```python
from build123d import *

# Parameters (mm, degrees)
BOSS_EXTRUDE2_DEPTH    = 6
FILLET1_R              = 1
LPATTERN1_COUNT        = 3
LPATTERN1_PITCH        = 37.5
FILLET1_OF_LPATTERN1_R = 1
SKETCH3_W              = 6
SKETCH3_H              = 12
BOSS_EXTRUDE3_DEPTH    = 6
SKETCH4_W              = 8
SKETCH4_H              = 6
CUT_EXTRUDE2_DEPTH     = 7
LPATTERN2_COUNT        = 2
LPATTERN2_PITCH        = 37.5
BOSS_EXTRUDE4_START    = -112.5
SKETCH3_2_W            = 6
SKETCH3_2_H            = 12
BOSS_EXTRUDE4_DEPTH    = 6
SKETCH5_W              = 6
SKETCH5_H              = 22.5
BOSS_EXTRUDE5_DEPTH    = 6


with BuildPart() as part:
    # Sketch2 → Boss-Extrude2 (new body)
    with BuildSketch(Plane(origin=(0, 0, 0), x_dir=(0, 0, -1), z_dir=(1, 0, 0))):
        Polygon((-18.75, 105.5), (-18.75, 89.5), (-18.75, -89.5), (18.75, -89.5), (18.75, 89.5), (18.75, 105.5), (12, 105.5), (11, 95.5), (4, 95.5), (4, 89.5), (-4, 89.5), (-4, 95.5), (-11, 95.5), (-12, 105.5), align=None)
    boss_extrude2 = extrude(amount=BOSS_EXTRUDE2_DEPTH)

    # Fillet1
    fillet1_edges = [part.edges().sort_by_distance(p)[0] for p in [
        (3, 95.5, -4),
        (3, 105.5, -12),
        (3, 105.5, 12),
        (3, 95.5, 4),
        (3, 89.5, 4),
        (3, 89.5, -4),
    ]]
    fillet(fillet1_edges, radius=FILLET1_R)

    # LPattern1: Boss-Extrude2 ×3
    with Locations(*[(0, 0, i * LPATTERN1_PITCH) for i in range(1, LPATTERN1_COUNT)]):
        add(boss_extrude2)

    # Fillet1 of LPattern1
    fillet1_of_lpattern1_edges = [part.edges().sort_by_distance(p)[0] for p in [
        (3, 95.5, 33.5),
        (3, 105.5, 25.5),
        (3, 105.5, 49.5),
        (3, 95.5, 41.5),
        (3, 89.5, 41.5),
        (3, 89.5, 33.5),
        (3, 95.5, 71),
        (3, 105.5, 63),
        (3, 105.5, 87),
        (3, 95.5, 79),
        (3, 89.5, 79),
        (3, 89.5, 71),
    ]]
    fillet(fillet1_of_lpattern1_edges, radius=FILLET1_OF_LPATTERN1_R)

    # Sketch3 → Boss-Extrude3 (add)
    with BuildSketch(Plane(origin=(0, 0, -18.75), x_dir=(-1, 0, 0), z_dir=(0, 0, -1))):
        with Locations((-3, 79.5)):
            Rectangle(SKETCH3_W, SKETCH3_H)
        with Locations((-3, -63.5)):
            Rectangle(SKETCH3_W, SKETCH3_H)
        with Locations((-3, 8)):
            Rectangle(SKETCH3_W, SKETCH3_H)
    extrude(amount=BOSS_EXTRUDE3_DEPTH)

    # Sketch4 → Cut-Extrude2 (cut, through all)
    with BuildSketch(Plane(origin=(0, 0, 0), x_dir=(0, 0, -1), z_dir=(1, 0, 0))):
        with Locations((-18.75, 86.5)):
            Rectangle(SKETCH4_W, SKETCH4_H)
    cut_extrude2 = extrude(amount=CUT_EXTRUDE2_DEPTH, mode=Mode.SUBTRACT)

    # LPattern2: Cut-Extrude2 ×2
    with Locations(*[(0, 0, i * LPATTERN2_PITCH) for i in range(1, LPATTERN2_COUNT)]):
        add(cut_extrude2, mode=Mode.SUBTRACT)

    # Sketch3_2 → Boss-Extrude4 (add)
    with BuildSketch(Plane(origin=(0, 0, -18.75), x_dir=(-1, 0, 0), z_dir=(0, 0, -1)).offset(BOSS_EXTRUDE4_START)):
        with Locations((-3, 79.5)):
            Rectangle(SKETCH3_2_W, SKETCH3_2_H)
        with Locations((-3, -63.5)):
            Rectangle(SKETCH3_2_W, SKETCH3_2_H)
        with Locations((-3, 8)):
            Rectangle(SKETCH3_2_W, SKETCH3_2_H)
    extrude(amount=-BOSS_EXTRUDE4_DEPTH)

    # Sketch5 → Boss-Extrude5 (add)
    with BuildSketch(Plane.XZ.offset(89.5)):
        with Locations((3, 15)):
            Rectangle(SKETCH5_W, SKETCH5_H)
        with Locations((3, 60)):
            Rectangle(SKETCH5_W, SKETCH5_H)
    extrude(amount=BOSS_EXTRUDE5_DEPTH)


solid = part.part
```
The listing builds one solid part. Answer for the finished solid, in the listing's coordinates (mm). A direction names the side the tool comes from. Give positions to 0.01 mm unless a question says otherwise; leave off trailing zeros. Write each loop counter-clockwise with the first axis right and the second up, starting at its lowest first coordinate (ties: lowest second). Pieces come first, ordered by that corner, then holes. Notation, with made-up numbers: (-29.5, 54) -> (-6.5, 54) arc R6 cw to (-6.5, 62) -> close; hole circle Ø6 at (-26, -6.5). An arc over 180 degrees is marked (long way). Use one line per item in the form item = value.
1) Section A-A on z = 56 is taken. Write down the section's boundary in (x, y), plus the area to 3 significant figures.
Result:
outline = (0, -95.5) -> (6, -95.5) -> (6, 83.5) -> (0, 83.5) -> close; (0, 89.5) -> (6, 89.5) -> (6, 105.5) -> (0, 105.5) -> close
area = 1,170 mm²
2) A tool of negligible diameter and unlimited length cuts with its end or side. For faces 4 (the flat face through (3, 105.5, -16)), 5 (the flat face through (3, -57.5, 97)), 6 (the flat face through (3, 83.5, 56)), 7 (the flat face through (2.96, 99.99, 48.95)), 8 (the flat face through (6, 6, 38)), from which of +Z, -Z, +X, -X, +Y, -Y can it reach the whole face along a straight path? Write none if from no direction.
Result:
face_4 = +Z, -Z, +X, -X, +Y
face_5 = +Z, +X, -X
face_6 = +X, -X
face_7 = +X, -X, +Y
face_8 = +Z, -Z, +X, +Y, -Y
3) Section B-B on x = 2.5 is taken. Count the separate pieces of the cut face and the enclosed holes in it, plus the area to 3 significant figures.
Result:
separate_pieces = 1
enclosed_holes = 2
area = 21,700 mm²
4) Each of these flat-tipped pins is pushed along its axis until it touches: P1, Ø2, axis at x = 4.5, y = -11.5, coming from the -Z side; P2, Ø3, axis at x = 1.5, z = 33.5, coming from the -Y side; P3, Ø1.5, axis at x = 2.5, y = -30.5, coming from the +Z side. Where does it stop, or does it pass through?
Result:
P1 = -18.75
P2 = -89.5
P3 = 93.75
5) Straight lines are drawn through the part: probe 1 along Y at (x, z) = (3.6, 59.5); probe 2 along Z at (x, y) = (1.8, 1); probe 3 along Y at (x, z) = (5.25, 44.5). For each, find the intervals that lie inside material, in ascending order.
Result:
probe_1 = -95.5 to 83.5, 89.5 to 105.5
probe_2 = -18.75 to 93.75
probe_3 = -89.5 to 95.5
6) Section C-C on y = 68 is taken. Write down the section's boundary in (x, z), plus the area to 3 significant figures.
Result:
outline = (0, -18.75) -> (6, -18.75) -> (6, 93.75) -> (0, 93.75) -> close
area = 675 mm²
7) Section D-D on z = -1 is taken. Write down the section's boundary in (x, y), plus the area to 3 significant figures.
Result:
outline = (0, -89.5) -> (6, -89.5) -> (6, 89.5) -> (0, 89.5) -> close
area = 1,070 mm²
8) For a pull along Z with two mould halves and no side action, classify faces 1 (the flat face through (3, -92, 3.75)), 2 (the flat face through (3, 14, -22)), 3 (the flat face through (3, 95.5, 45)) as +Z half, -Z half, draft (parallel to the pull), parting line (faces both ways), or undercut.
Result:
face_1 = -Z half
face_2 = draft
face_3 = undercut
